Could you check a few things on this model? Use its own coordinates, in mm. A direction names the side the tool comes from. Coordinates: 2 decimals unless noted, no trailing zeros. Loops run counter-clockwise (first coordinate to the right, second up) from the corner with the lowest first, then second, coordinate; pieces in that order, holes last. Notation, with made-up numbers: M 63.25,32 L 107.25,32 A30 cw 107.25,62 Z; hole C 32,-11 d3. An arc over 180 degrees is marked long. Return JSON: item names as keys, results as strings. Group by question number.
from build123d import *

# Parameters (mm, degrees)
SKETCH1_R           = 1.5
SKETCH1_R_2         = 20
BOSS_EXTRUDE1_DEPTH = 3
SKETCH2_R           = 24
SKETCH2_R_2         = 20
BOSS_EXTRUDE2_DEPTH = 40
SKETCH3_R           = 24
BOSS_EXTRUDE3_DEPTH = 3
SKETCH4_R           = 13.5
CUT_EXTRUDE1_DEPTH  = 67.034082109
SKETCH5_R           = 15.5
SKETCH5_R_2         = 13.5
BOSS_EXTRUDE4_DEPTH = 4
FILLET1_R           = 1
FILLET2_R           = 2


with BuildPart() as part:
    # Sketch1 → Boss-Extrude1 (new body)
    with BuildSketch(Plane(origin=(0, 0, 0), x_dir=(1, 0, 0), z_dir=(0, 1, 0))):
        with BuildLine():
            ThreePointArc((-29.774250944, 3.673415402), (-29.785177171, 3.58374398), (-29.795833333, 3.494040065))
            ThreePointArc((-29.795833333, 3.494040065), (-33.5, 0), (-29.795833333, -3.494040065))
            Line((-29.795833333, -3.494040065), (-23.744297927, -3.494040065))
            ThreePointArc((-23.744297927, -3.494040065), (-16.972692501, -16.968432728), (-3.5, -23.743420141))
            Line((-3.5, -23.743420141), (-3.5, -29.795133831))
            ThreePointArc((-3.5, -29.795133831), (-3.49702005, -29.795483731), (-3.494040065, -29.795833333))
            ThreePointArc((-3.494040065, -29.795833333), (0, -33.5), (3.494040064, -29.795833333))
            Line((3.494040064, -29.795833333), (3.494040064, -23.744297927))
            ThreePointArc((3.494040064, -23.744297927), (16.970562748, -16.970562749), (23.744297927, -3.494040065))
            Line((23.744297927, -3.494040065), (29.795833333, -3.494040065))
            ThreePointArc((29.795833333, -3.494040064), (33.5, 0), (29.795833333, 3.494040064))
            Line((29.795833333, 3.494040064), (23.741608141, 3.512270334))
            ThreePointArc((23.741608141, 3.512270334), (16.964046346, 16.97707665), (3.494040064, 23.744297927))
            Line((3.494040064, 23.744297927), (3.494040064, 29.795833333))
            ThreePointArc((3.494040064, 29.795833333), (0, 33.5), (-3.494040065, 29.795833333))
            ThreePointArc((-3.494040064, 29.795833333), (-3.49702005, 29.795483731), (-3.5, 29.795133831))
            Line((-3.5, 29.795133831), (-3.5, 23.743420141))
            ThreePointArc((-3.5, 23.743420141), (-16.914985868, 17.025958213), (-23.720025751, 3.655185133))
            Line((-23.720025751, 3.655185133), (-29.774250944, 3.673415402))
        make_face()
        with Locations(Location((0, -30, 0), (0, 0, 270))):
            Circle(SKETCH1_R, mode=Mode.SUBTRACT)
        with Locations(Location((-30, 0, 0), (0, 0, 270))):
            Circle(SKETCH1_R, mode=Mode.SUBTRACT)
        with Locations(Location((0, 0, 0), (0, 0, 270))):
            Circle(SKETCH1_R_2, mode=Mode.SUBTRACT)
        with Locations(Location((0, 30, 0), (0, 0, 270))):
            Circle(SKETCH1_R, mode=Mode.SUBTRACT)
        with Locations(Location((30, 0, 0), (0, 0, 270))):
            Circle(SKETCH1_R, mode=Mode.SUBTRACT)
    extrude(amount=BOSS_EXTRUDE1_DEPTH)

    # Sketch2 → Boss-Extrude2 (add)
    with BuildSketch(Plane(origin=(0, 3, 0), x_dir=(1, 0, 0), z_dir=(0, 1, 0))):
        with Locations(Location((0, 0, 0), (0, 0, 81.628843141))):
            Circle(SKETCH2_R)
        with Locations(Location((0, 0, 0), (0, 0, 270))):
            Circle(SKETCH2_R_2, mode=Mode.SUBTRACT)
    extrude(amount=BOSS_EXTRUDE2_DEPTH)

    # Sketch3 → Boss-Extrude3 (add)
    with BuildSketch(Plane(origin=(0, 43, 0), x_dir=(1, 0, 0), z_dir=(0, 1, 0))):
        with Locations(Location((0, 0, 0), (0, 0, 81.628843141))):
            Circle(SKETCH3_R)
    extrude(amount=BOSS_EXTRUDE3_DEPTH)

    # Sketch4 → Cut-Extrude1 (cut, through all)
    with BuildSketch(Plane(origin=(0, 46, 0), x_dir=(1, 0, 0), z_dir=(0, 1, 0))):
        with Locations(Location((0, 0, 0), (0, 0, 270))):
            Circle(SKETCH4_R)
    extrude(amount=-CUT_EXTRUDE1_DEPTH, mode=Mode.SUBTRACT)

    # Sketch5 → Boss-Extrude4 (add)
    with BuildSketch(Plane.XZ.offset(-43)):
        with Locations(Location((0, 0, 0), (0, 0, 90))):
            Circle(SKETCH5_R)
        with Locations(Location((0, 0, 0), (0, 0, 90))):
            Circle(SKETCH5_R_2, mode=Mode.SUBTRACT)
    extrude(amount=BOSS_EXTRUDE4_DEPTH)

    # Fillet1
    fillet1_edges = [part.edges().sort_by_distance(p)[0] for p in [
        (0, 43, -15.5),
    ]]
    fillet(fillet1_edges, radius=FILLET1_R)

    # Fillet2
    fillet2_edges = [part.edges().sort_by_distance(p)[0] for p in [
        (0, 39, -13.5),
    ]]
    fillet(fillet2_edges, radius=FILLET2_R - 0.0001)  # a hair under: the kernel refuses the full size


solid = part.part
(1) We'd pull the mould along Z, two halves only. Please class faces 5 (the face through (-28, 3, 0)), 6 (the face through (0.07, 1.48, -31.5)), 7 (the face through (-33.5, 1.5, -0.1)): +Z half, -Z half, draft (parallel to the pull), parting line (faces both ways), or undercut.
(2) Imagine slicing it at D-D, the plane z = 22. Write out the boundary of the cut face in (x, y), then the cut area to 3 significant figures.
(3) Will these pins go through, and if not, where does the flat tip stop? P1, Ø3.5, axis at y = 2, z = -26, coming from the +X side; P2, Ø1, axis at y = 5.5, z = 8.5, coming from the -X side; P3, Ø2, axis at x = -27.5, z = 1.5, coming from the +Y side.
(4) If I drill on L1, parallel to X at y = 1.25, z = -30; L2, parallel to Z at x = 0, y = 44.35; L3, parallel to X at y = 2, z = 0, over which ranges is the centre line in solid material (lowest first)? Write a range as [from, to].
(5) Imagine slicing it at C-C, the plane y = 36.5. Write out the boundary of the cut face in (x, z), then the cut area to 3 significant figures.
(6) Imagine slicing it at A-A, the plane z = 0. Count the separate pieces of the cut face and the enclosed holes in it, then the cut area to 3 significant figures.
(7) For faces 1 (the face through (-16, 43, -5)), 2 (the face through (3.494, 1, 27)), 3 (the face through (-3.5, 1, 27)), 4 (the face through (3.494, 1, -27)), which set-ups out of +Z, -Z, +X, -X, +Y, -Y let a thin tool reach every point of the face, with its end or its side?
Checks:
{
 "1": {"face 5": "draft", "face 6": "undercut", "face 7": "parting line"},
 "2": {"outline": "M -9.59,0 L 9.59,0 L 9.59,46 L -9.59,46 Z", "area": "882 mm²"},
 "3": {"P1": "x = 3.49", "P2": "x = -22.63", "P3": "y = 3"},
 "4": {"L1": "[-3.5, -1.5], [1.5, 3.5]", "L2": "[-24, -13.5], [13.5, 24]", "L3": "[-33.5, -31.5], [-28.5, -20], [20, 28.5], [31.5, 33.5]"},
 "5": {"outline": "C 0,0 d48; hole C 0,0 d40", "area": "553 mm²"},
 "6": {"separate pieces": "4", "enclosed holes": "0", "area": "461 mm²"},
 "7": {"face 1": "-Y", "face 2": "+Z, +X, +Y, -Y", "face 3": "+Z, -X, +Y, -Y", "face 4": "-Z, +X, +Y, -Y"}
}
